from build123d import *

# Parameters (mm, degrees)
CROQUIS1_R              = 29
CROQUIS1_R_2            = 20
SALIENTE_EXTRUIR1_DEPTH = 9
CORTAR_EXTRUIR1_REACH   = 43.988
CROQUIS2_W              = 6
CROQUIS2_H              = 2.5
CROQUIS2_W_2            = 2.5
CROQUIS2_H_2            = 6


with BuildPart() as part:
    # Croquis1 → Saliente-Extruir1 (new body)
    with BuildSketch(Plane(origin=(0, 0, 0), x_dir=(1, 0, 0), z_dir=(0, 1, 0))):
        with Locations(Location((0, 0, 0), (0, 0, 270))):
            Circle(CROQUIS1_R)
        with Locations(Location((0, 0, 0), (0, 0, 270))):
            Circle(CROQUIS1_R_2, mode=Mode.SUBTRACT)
    extrude(amount=SALIENTE_EXTRUIR1_DEPTH)

    # Croquis2 → Cortar-Extruir1 (cut, up to next)
    with BuildSketch(Plane(origin=(0, 9, 0), x_dir=(1, 0, 0), z_dir=(0, 1, 0)), mode=Mode.PRIVATE) as cortar_extruir1_sk1:
        with Locations((0, 27.75)):
            Rectangle(CROQUIS2_W, CROQUIS2_H)
    cortar_extruir1_tool1 = extrude(cortar_extruir1_sk1.sketch, amount=-CORTAR_EXTRUIR1_REACH, mode=Mode.PRIVATE) & part.part
    # Croquis2 → Cortar-Extruir1 (cut, up to next)
    with BuildSketch(Plane(origin=(0, 9, 0), x_dir=(1, 0, 0), z_dir=(0, 1, 0)), mode=Mode.PRIVATE) as cortar_extruir1_sk2:
        with Locations((0, -27.75)):
            Rectangle(CROQUIS2_W, CROQUIS2_H)
    cortar_extruir1_tool2 = extrude(cortar_extruir1_sk2.sketch, amount=-CORTAR_EXTRUIR1_REACH, mode=Mode.PRIVATE) & part.part
    # Croquis2 → Cortar-Extruir1 (cut, up to next)
    with BuildSketch(Plane(origin=(0, 9, 0), x_dir=(1, 0, 0), z_dir=(0, 1, 0)), mode=Mode.PRIVATE) as cortar_extruir1_sk3:
        with Locations((27.75, 0)):
            Rectangle(CROQUIS2_W_2, CROQUIS2_H_2)
    cortar_extruir1_tool3 = extrude(cortar_extruir1_sk3.sketch, amount=-CORTAR_EXTRUIR1_REACH, mode=Mode.PRIVATE) & part.part
    # Croquis2 → Cortar-Extruir1 (cut, up to next)
    with BuildSketch(Plane(origin=(0, 9, 0), x_dir=(1, 0, 0), z_dir=(0, 1, 0)), mode=Mode.PRIVATE) as cortar_extruir1_sk4:
        with Locations((-27.75, 0)):
            Rectangle(CROQUIS2_W_2, CROQUIS2_H_2)
    cortar_extruir1_tool4 = extrude(cortar_extruir1_sk4.sketch, amount=-CORTAR_EXTRUIR1_REACH, mode=Mode.PRIVATE) & part.part
    add(cortar_extruir1_tool1.solids().sort_by_distance((0, 9, -27.75))[0], mode=Mode.SUBTRACT)
    add(cortar_extruir1_tool2.solids().sort_by_distance((0, 9, 27.75))[0], mode=Mode.SUBTRACT)
    add(cortar_extruir1_tool3.solids().sort_by_distance((27.75, 9, 0))[0], mode=Mode.SUBTRACT)
    add(cortar_extruir1_tool4.solids().sort_by_distance((-27.75, 9, 0))[0], mode=Mode.SUBTRACT)

    # Croquis3 → Cortar-Revolución1 (revolve, cut)
    with BuildSketch(Plane(origin=(0, 0, 0), x_dir=(0, 0, -1), z_dir=(1, 0, 0)), mode=Mode.PRIVATE) as cortar_revoluci_n1_sk:
        Polygon((-29, 9), (-25, 9), (-29, 6.690598923), align=None)
    revolve(cortar_revoluci_n1_sk.sketch.rotate(Axis((0, 9, 0), (0, -1, 0)), 185.937772452), axis=Axis((0, 9, 0), (0, -1, 0)), mode=Mode.SUBTRACT)


solid = part.part
Model file for the job. Use its own axes, mm. A direction names the side the tool comes from. Round coordinates to 2 decimals unless told otherwise and drop trailing zeros. Order: outer loops, then holes, each group sorted by start corner. A loop starts at its lowest first (then second) coordinate and runs counter-clockwise, first axis right, second up.
(1) Band-saw the part on A-A (z = 0). List the corners of the cut face in (x, y).
(2) Band-saw the part on C-C (y = 2.5). List the corners of the cut face in (x, z).
(3) Pin check, flat tips, straight feed: pin 1 (1.2 mm diameter, centred on y = 3, z = 27, fed in from +X); pin 2 (0.7 mm diameter, centred on y = 3, z = -27, fed in from +X); pin 3 (1.5 mm diameter, centred on x = 6.5, y = 5, fed in from -Z); pin 4 (1.5 mm diameter, centred on y = 6.5, z = 2.5, fed in from +X). Stop position of each tip, or through.
(4) Pull direction X, two halves, no side cores. Call faces 1 (the face through (-26.5, 4, 0)), 2 (the face through (28, 4, -3)), 3 (the face through (0, 4, -26.5)): released by +X, released by -X, zero draft, split by the parting line, or undercut.
(5) Drill centre lines: line 1 (X direction, y = 6.25, z = 0); line 2 (Z direction, x = 0.5, y = 2.75); line 3 (Z direction, x = 6, y = 7.5). Where is each one in solid material? Low to high.
(6) 3-axis set-ups, long thin cutter, end or side, ignore diameter. For faces 4 (the face through (26.5, 4, 0)), 5 (the face through (0, 4, 26.5)), 6 (the face through (3, 4, -28)), 7 (the face through (-28, 4, 3)), 8 (the face through (10.035, 8.856, -23.17)): which of +Z, -Z, +X, -X, +Y, -Y reach the whole face in a straight line?
(7) Band-saw the part on B-B (x = 0). List the corners of the cut face in (y, z).
Verdict:
1. outline: (-26.5, 0) - (-20, 0) - (-20, 9) - (-25, 9) - (-26.5, 8.13) - close; (20, 0) - (26.5, 0) - (26.5, 8.13) - (25, 9) - (20, 9) - close
2. outline: (-28.84, -3) arc R29 ccw to (-3, -28.84) - (-3, -26.5) - (3, -26.5) - (3, -28.84) arc R29 ccw to (28.84, -3) - (26.5, -3) - (26.5, 3) - (28.84, 3) arc R29 ccw to (3, 28.84) - (3, 26.5) - (-3, 26.5) - (-3, 28.84) arc R29 ccw to (-28.84, 3) - (-26.5, 3) - (-26.5, -3) - close; hole circle Ø40 at (0, 0)
3. pin 1: stops at x = 12
3. pin 2: stops at x = 11.44
3. pin 3: stops at z = -28.42
3. pin 4: stops at x = 28.84
4. face 1: released by -X
4. face 2: zero draft
4. face 3: undercut
5. line 1: x = -26.5 to -20, 20 to 26.5
5. line 2: z = -26.5 to -19.99, 19.99 to 26.5
5. line 3: z = -26.94 to -19.08, 19.08 to 26.94
6. face 4: +X, +Y, -Y
6. face 5: +Z, +Y, -Y
6. face 6: -Z, +Y, -Y
6. face 7: -X, +Y, -Y
6. face 8: +Y
7. outline: (0, -26.5) - (8.13, -26.5) - (9, -25) - (9, -20) - (0, -20) - close; (0, 20) - (9, 20) - (9, 25) - (8.13, 26.5) - (0, 26.5) - close
